Can you work these out from the model? Positions are in its coordinate system, mm. A direction names the side the tool comes from. Round coordinates to 2 decimals unless told otherwise and drop trailing zeros. Write each loop counter-clockwise with the first axis right and the second up, starting at its lowest first coordinate (ties: lowest second). Pieces come first, ordered by that corner, then holes. Notation, with made-up numbers: M 22.5,38.5 L 55.5,38.5 A17 ccw 55.5,61.5 Z; hole C -8.75,3.25 d10. An arc over 180 degrees is marked long. Answer as a JSON object with one key per item and string values. Group by question number.
1) Please list where these lines run through material, in increasing order: L1, parallel to Y at x = 0, z = 1.75; L2, parallel to Y at x = 0, z = 7.3; L3, parallel to X at y = 0, z = 5.75. Write a range as [from, to].
2) Suppose I cut it at C-C, the plane z = 3.5. Write out the boundary of the cut face in (x, y), and give its area (3 significant figures).
3) Suppose I cut it at B-B, the plane x = 0. Write out the boundary of the cut face in (y, z), and give its area (3 significant figures).
4) On a 3-axis mill with a long thin cutter (end or side, diameter ignored), from which of +Z, -Z, +X, -X, +Y, -Y can I reach the whole of each face in a straight line? I mean faces 4 (the flat face through (-2.5, 2.2, 4)), 5 (the flat face through (0, -2, 0)). Say none if no direction works.
5) I'm going to push flat-ended pins straight in: pin 1 Ø4 at (y, z) = (0, 3.5) entering from +X; pin 2 Ø1.5 at (x, z) = (2, 1.5) entering from -Y; pin 3 Ø5 at (x, y) = (-4, -2) entering from +Z; pin 4 Ø2 at (y, z) = (1, 8) entering from +X. Where does each tip first touch, or does it pass through?
6) If we mould it in two halves opening along X, with no side actions, what happens to faces 1 (the cylindrical face through (-2.4, 1.8, 2)), 2 (the cylindrical face through (0, 1, 7)), 3 (the flat face through (4.27, 2.6, 5.26))? For each: +X half, -X half, draft (parallel to the pull), parting line (faces both ways), or undercut.
from build123d import *

# Parameters (mm, degrees)
F1_DEPTH = 10
F2_W     = 4.670898
F2_H     = 6.321549
F4_R     = 0.2
F5_DEPTH = 10.001


with BuildPart() as f1:
    # F0 (on Top) → F1 (new body)
    with BuildSketch(Plane.XY):
        Polygon((5.770634, 0.18198), (2.727718, 5.088505), (-3.042916, 4.906526), (-5.770634, -0.18198), (-2.727718, -5.088505), (3.042916, -4.906526), align=None)
    extrude(amount=F1_DEPTH)

    # F2 (on Front) → F3 (revolve, cut)
    with BuildSketch(Plane.XZ):
        with Locations((5.335449, 0.839225)):
            Rectangle(F2_W, F2_H)
        Polygon((0.4, 10.880456), (0.4, 10.104967), (5.705611, 6), (7.525738, 6), (7.525738, 10.880456), align=None)
        Polygon((0, 9), (0, -1.974234), (1.75, -1.974234), (1.75, 4.5), (1, 5), (1, 8), align=None)
    revolve(axis=Axis((0, 0, 3.313374), (0, 0, -1)), mode=Mode.SUBTRACT)

    # F4 (on face) → F5 (cut, through all)
    with BuildSketch(Plane.XY.offset(10)):
        Circle(F4_R)
    extrude(amount=-F5_DEPTH, mode=Mode.SUBTRACT)


solid = f1.part
Results:
{
 "1": {"L1": "[-3, -1.75], [1.75, 3]", "L2": "[-4.03, -1], [1, 4.03]", "L3": "[-5.67, -1], [1, 5.67]"},
 "2": {"outline": "C 0,0 d6; hole C 0,0 d3.5", "area": "18.7 mm^2"},
 "3": {"outline": "M -5,4 L -3,4 L -3,0 L -1.75,0 L -1.75,4.5 L -1,5 L -1,8 L -0.2,8.8 L -0.2,10 L -0.54,10 L -5,6.54 Z; M 0.2,8.8 L 1,8 L 1,5 L 1.75,4.5 L 1.75,0 L 3,0 L 3,4 L 5,4 L 5,6.54 L 0.54,10 L 0.2,10 Z", "area": "44.0 mm^2"},
 "4": {"face 4": "-Z", "face 5": "-Z, +X, -X, +Y, -Y"},
 "5": {"pin 1": "x = 5.77", "pin 2": "y = -2.73", "pin 3": "z = 8.89", "pin 4": "x = 4.32"},
 "6": {"face 1": "parting line", "face 2": "undercut", "face 3": "+X half"}
}
